from build123d import *

# Parameters (mm, degrees)
SKETCH1_R           = 13.918584035
BOSS_EXTRUDE1_DEPTH = 63.5
BOSS_EXTRUDE2_START = -3.81
SKETCH3_R           = 20.776584035
SKETCH3_R_2         = 13.918584035
BOSS_EXTRUDE2_DEPTH = 3.81
FILLET1_R           = 15.24
SKETCH4_R           = 20.776584035
SKETCH4_R_2         = 13.918584035
BOSS_EXTRUDE3_DEPTH = 3.81
FILLET2_R           = 15.24
SKETCH7_R           = 1.27
CUT_EXTRUDE1_DEPTH  = 419.299996556


with BuildPart() as part:
    # Sketch1 → Boss-Extrude1 (new, symmetric)
    with BuildSketch(Plane(origin=(0, 0, 0), x_dir=(0, 0, -1), z_dir=(1, 0, 0))):
        with Locations((364.49, 81.28)):
            Circle(SKETCH1_R)
    extrude(amount=BOSS_EXTRUDE1_DEPTH, both=True)

    # Sketch3 → Boss-Extrude2 (add)
    with BuildSketch(Plane.ZY.offset(63.5).offset(BOSS_EXTRUDE2_START)):
        with Locations((-364.49, 81.28)):
            Circle(SKETCH3_R)
        with Locations((-364.49, 81.28)):
            Circle(SKETCH3_R_2, mode=Mode.SUBTRACT)
    extrude(amount=BOSS_EXTRUDE2_DEPTH)

    # Fillet1
    # the kernel refuses this fillet: 15.24 mm, written as the material it adds along each edge
    with BuildSketch(Plane(origin=(-59.69, 81.28, -364.49), x_dir=(0, 0, -1), z_dir=(0, -1, 0))) as fillet1_piece_1:
        with BuildLine():
            CenterArc((29.158584035, 12.727909333), FILLET1_R, 180, 56.632987031)
            Line((20.776584035, 0), (20.608944035, -0.254558187))
            ThreePointArc((20.608944035, -0.254558187), (17.347584035, -0.3048), (13.918584035, -0.3048))
            Line((13.918584035, -0.3048), (13.613784035, 0))
            Line((13.613784035, 0), (13.613784035, 12.727909333))
            Line((13.613784035, 12.727909333), (13.918584035, 12.727909333))
        make_face()
    revolve(axis=Axis((-59.69, 81.28, -364.49), (1, 0, 0)))

    # Sketch4 → Boss-Extrude3 (add)
    with BuildSketch(Plane(origin=(63.5, 0, 0), x_dir=(0, 0, -1), z_dir=(1, 0, 0))):
        with Locations(Location((364.49, 81.28, 0), (0, 0, 180))):
            Circle(SKETCH4_R)
        with Locations(Location((364.49, 81.28, 0), (0, 0, 180))):
            Circle(SKETCH4_R_2, mode=Mode.SUBTRACT)
    extrude(amount=-BOSS_EXTRUDE3_DEPTH)

    # Fillet2
    # the kernel refuses this fillet: 15.24 mm, written as the material it adds along each edge
    with BuildSketch(Plane(origin=(59.69, 81.28, -364.49), x_dir=(0, 0, -1), z_dir=(0, 1, 0))) as fillet2_piece_1:
        with BuildLine():
            CenterArc((29.158584035, 12.727909333), FILLET2_R, 180, 56.632987031)
            Line((20.776584035, 0), (20.608944035, -0.254558187))
            ThreePointArc((20.608944035, -0.254558187), (17.347584035, -0.3048), (13.918584035, -0.3048))
            Line((13.918584035, -0.3048), (13.613784035, 0))
            Line((13.613784035, 0), (13.613784035, 12.727909333))
            Line((13.613784035, 12.727909333), (13.918584035, 12.727909333))
        make_face()
    revolve(axis=Axis((59.69, 81.28, -364.49), (-1, 0, 0)))

    # Sketch7 → Cut-Extrude1 (cut, through all)
    with BuildSketch(Plane(origin=(63.5, 0, 0), x_dir=(0, 0, -1), z_dir=(1, 0, 0))):
        with Locations((372.408936292, 81.28)):
            Circle(SKETCH7_R)
        with Locations((368.449468146, 88.138)):
            Circle(SKETCH7_R)
        with Locations((360.530531854, 88.138)):
            Circle(SKETCH7_R)
        with Locations((356.571063708, 81.28)):
            Circle(SKETCH7_R)
        with Locations((360.530531854, 74.422)):
            Circle(SKETCH7_R)
        with Locations((368.449468146, 74.422)):
            Circle(SKETCH7_R)
        Polygon((372.408936292, 81.28), (368.449468146, 88.138), (360.530531854, 88.138), (356.571063708, 81.28), (360.530531854, 74.422), (368.449468146, 74.422), align=None)
        with BuildLine():
            ThreePointArc((359.895531854, 87.038147737), (361.165531854, 87.038147737), (361.800531854, 88.138))
            Line((361.800531854, 88.138), (360.530531854, 88.138))
            Line((360.530531854, 88.138), (359.895531854, 87.038147737))
        make_face()
        with BuildLine():
            Line((360.530531854, 88.138), (361.800531854, 88.138))
            ThreePointArc((361.800531854, 88.138), (359.895531854, 89.237852263), (359.895531854, 87.038147737))
            Line((359.895531854, 87.038147737), (360.530531854, 88.138))
        make_face()
        with BuildLine():
            ThreePointArc((357.841063708, 81.28), (357.670915971, 81.915), (357.206063708, 82.379852263))
            Line((357.206063708, 82.379852263), (356.571063708, 81.28))
            Line((356.571063708, 81.28), (357.206063708, 80.180147737))
            ThreePointArc((357.206063708, 80.180147737), (357.670915971, 80.645), (357.841063708, 81.28))
        make_face()
        with BuildLine():
            Line((356.571063708, 81.28), (357.206063708, 82.379852263))
            ThreePointArc((357.206063708, 82.379852263), (355.301063708, 81.28), (357.206063708, 80.180147737))
            Line((357.206063708, 80.180147737), (356.571063708, 81.28))
        make_face()
        with BuildLine():
            ThreePointArc((359.895531854, 75.521852263), (359.895531854, 73.322147737), (361.800531854, 74.422))
            Line((361.800531854, 74.422), (360.530531854, 74.422))
            Line((360.530531854, 74.422), (359.895531854, 75.521852263))
        make_face()
        with BuildLine():
            Line((360.530531854, 74.422), (361.800531854, 74.422))
            ThreePointArc((361.800531854, 74.422), (361.165531854, 75.521852263), (359.895531854, 75.521852263))
            Line((359.895531854, 75.521852263), (360.530531854, 74.422))
        make_face()
        with BuildLine():
            ThreePointArc((367.179468146, 88.138), (367.814468146, 87.038147737), (369.084468146, 87.038147737))
            Line((369.084468146, 87.038147737), (368.449468146, 88.138))
            Line((368.449468146, 88.138), (367.179468146, 88.138))
        make_face()
        with BuildLine():
            Line((368.449468146, 88.138), (369.084468146, 87.038147737))
            ThreePointArc((369.084468146, 87.038147737), (369.549320409, 87.503), (369.719468146, 88.138))
            ThreePointArc((369.719468146, 88.138), (368.449468146, 89.408), (367.179468146, 88.138))
            Line((367.179468146, 88.138), (368.449468146, 88.138))
        make_face()
        with BuildLine():
            Line((371.773936292, 80.180147737), (372.408936292, 81.28))
            Line((372.408936292, 81.28), (371.773936292, 82.379852263))
            ThreePointArc((371.773936292, 82.379852263), (371.138936292, 81.28), (371.773936292, 80.180147737))
        make_face()
        with BuildLine():
            Line((371.773936292, 82.379852263), (372.408936292, 81.28))
            Line((372.408936292, 81.28), (371.773936292, 80.180147737))
            ThreePointArc((371.773936292, 80.180147737), (373.043936292, 80.180147737), (373.678936292, 81.28))
            ThreePointArc((373.678936292, 81.28), (373.043936292, 82.379852263), (371.773936292, 82.379852263))
        make_face()
        with BuildLine():
            ThreePointArc((369.719468146, 74.422), (369.549320409, 75.057), (369.084468146, 75.521852263))
            Line((369.084468146, 75.521852263), (368.449468146, 74.422))
            Line((368.449468146, 74.422), (367.179468146, 74.422))
            ThreePointArc((367.179468146, 74.422), (368.449468146, 73.152), (369.719468146, 74.422))
        make_face()
        with BuildLine():
            Line((368.449468146, 74.422), (369.084468146, 75.521852263))
            ThreePointArc((369.084468146, 75.521852263), (367.814468146, 75.521852263), (367.179468146, 74.422))
            Line((367.179468146, 74.422), (368.449468146, 74.422))
        make_face()
    extrude(amount=-CUT_EXTRUDE1_DEPTH, mode=Mode.SUBTRACT)


solid = part.part
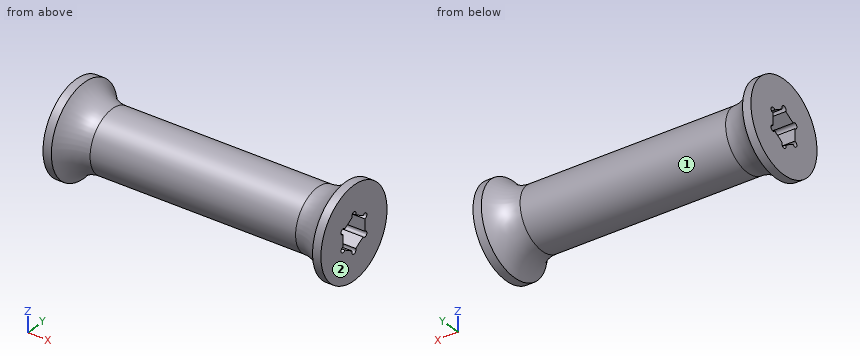
Work out the finished part from the listing and answer in its coordinate system (mm). Face numbers are marked on the shaded views. A direction names the side the tool comes from. Round coordinates to 2 decimals unless told otherwise and drop trailing zeros. Write each loop counter-clockwise with the first axis right and the second up, starting at its lowest first coordinate (ties: lowest second). Pieces come first, ordered by that corner, then holes. Notation, with made-up numbers: (-35.75, 15.5) - (-2.75, 15.5) arc R27 ccw to (-2.75, 43.5) - close; hole circle Ø4 at (55.5, 28.25). An arc over 180 degrees is marked (long way). Answer in a Markdown table with one row per item. Add a question column.
1. A cutting plane is placed at B-B, the plane x = 18.5. Determine the outline of the cut face in (y, z), and give its area (3 significant figures).
2. A cutting plane is placed at C-C, the plane x = 50.5. Determine the outline of the cut face in (y, z).
3. A cutting plane is placed at A-A, the plane z = -364.49. Determine the outline of the cut face in (x, y).
4. For the marked faces 1 and 2, determine the directions among +Z, -Z, +X, -X, +Y, -Y from which every point of the face is accessible in a straight line to the end or side of a thin tool.
5. Find the intervals of material crossed by line 1 along X through (y, z) = (88, -381); line 2 along Y through (x, z) = (-21, -371); line 3 along Z through (x, y) = (24.5, 86), in increasing order. Write a range as from..to.
6. Given pin 1 (2 mm diameter, centred on y = 73.5, z = -369, fed in from +X); pin 2 (3 mm diameter, centred on x = 30.5, z = -365.5, fed in from -Y); pin 3 (2 mm diameter, centred on y = 81.28, z = -372.41, fed in from -X); pin 4 (1.6 mm diameter, centred on x = 4.5, z = -365.5, fed in from +Y), each flat-ended and moving along its own axis, determine where each tip first touches the part or whether it passes through.
Worked out:
| question | item | result |
|---|---|---|
| 1 | outline | circle Ø27.84 at (81.28, -364.49); hole (74.42, -367.18) arc R1.27 ccw (long way) to (75.52, -369.08) - (80.18, -371.77) arc R1.27 ccw (long way) to (82.38, -371.77) - (87.04, -369.08) arc R1.27 ccw (long way) to (88.14, -367.18) - (88.14, -361.8) arc R1.27 ccw (long way) to (87.04, -359.9) - (82.38, -357.21) arc R1.27 ccw (long way) to (80.18, -357.21) - (75.52, -359.9) arc R1.27 ccw (long way) to (74.42, -361.8) - close |
| 1 | area | 425 mm^2 |
| 2 | outline | circle Ø28.67 at (81.28, -364.49); hole (74.42, -367.18) arc R1.27 ccw (long way) to (75.52, -369.08) - (80.18, -371.77) arc R1.27 ccw (long way) to (82.38, -371.77) - (87.04, -369.08) arc R1.27 ccw (long way) to (88.14, -367.18) - (88.14, -361.8) arc R1.27 ccw (long way) to (87.04, -359.9) - (82.38, -357.21) arc R1.27 ccw (long way) to (80.18, -357.21) - (75.52, -359.9) arc R1.27 ccw (long way) to (74.42, -361.8) - close |
| 3 | outline | (-63.5, 60.5) - (-59.69, 60.5) arc R15.24 cw to (-46.96, 67.36) - (46.96, 67.36) arc R15.24 cw to (59.69, 60.5) - (63.5, 60.5) - (63.5, 74.42) - (-63.5, 74.42) - close; (-63.5, 88.14) - (63.5, 88.14) - (63.5, 102.06) - (59.69, 102.06) arc R15.24 cw to (46.96, 95.2) - (-46.96, 95.2) arc R15.24 cw to (-59.69, 102.06) - (-63.5, 102.06) - close |
| 4 | face 1 | none |
| 4 | face 2 | +Z, -Z, +X, +Y, -Y |
| 5 | line 1 | -63.5..-57.15, 57.15..63.5 |
| 5 | line 2 | 68.98..78.84, 83.72..93.58 |
| 5 | line 3 | -377.58..-369.68, -359.3..-351.4 |
| 6 | pin 1 | x = 63.5 |
| 6 | pin 2 | y = 67.36 |
| 6 | pin 3 | through |
| 6 | pin 4 | y = 95.2 |
